```python
from build123d import *

# Parameters (mm, degrees)
SKETCH1_W                                  = 100
SKETCH1_H                                  = 100
BOSS_EXTRUDE1_DEPTH                        = 15
SKETCH2_R                                  = 0.5
CUT_EXTRUDE1_DEPTH                         = 2
MIRROR1_AT_THE_SECOND_PLANE_COPY_1_SKETC_R = 0.5
MIRROR1_AT_THE_SECOND_PLANE_COPY_1_DEPTH   = 2


with BuildPart() as part:
    # Sketch1 → Boss-Extrude1 (new body, symmetric)
    with BuildSketch(Plane(origin=(0, 0, 0), x_dir=(1, 0, 0), z_dir=(0, 1, 0))):
        Rectangle(SKETCH1_W, SKETCH1_H)
    extrude(amount=BOSS_EXTRUDE1_DEPTH, both=True)

    # Sketch2 → Cut-Extrude1 (cut)
    with BuildSketch(Plane(origin=(0, 15, 0), x_dir=(1, 0, 0), z_dir=(0, 1, 0))):
        Circle(SKETCH2_R)
        with BuildLine():
            Line((-28.090825198, -33.465171233), (-27.090825198, -33.120843619))
            ThreePointArc((-27.090825198, -33.120843619), (-25.819738468, -33.740794041), (-26.439688889, -35.011880771))
            Line((-26.439688889, -35.011880771), (-27.439688889, -35.356208384))
            ThreePointArc((-27.439688889, -35.356208384), (-28.710775619, -34.736257963), (-28.090825198, -33.465171233))
        make_face()
    cut_extrude1 = extrude(amount=-CUT_EXTRUDE1_DEPTH, mode=Mode.SUBTRACT)

    # Mirror1: Cut-Extrude1 across plane
    add(cut_extrude1.mirror(Plane.XY), mode=Mode.SUBTRACT)

    # Mirror1 at the second plane: Cut-Extrude1 across plane
    add(cut_extrude1.mirror(Plane(origin=(0, 0, 0), x_dir=(0, 0, 1), z_dir=(1, 0, 0))), mode=Mode.SUBTRACT)

    # Mirror1 at the second plane copy 1 sketc → Mirror1 at the second plane copy 1 (cut)
    with BuildSketch(Plane(origin=(0, 15, 0), x_dir=(-1, 0, 0), z_dir=(0, 1, 0))):
        Circle(MIRROR1_AT_THE_SECOND_PLANE_COPY_1_SKETC_R)
        with BuildLine():
            Line((-28.090825198, -33.465171233), (-27.090825198, -33.120843619))
            ThreePointArc((-27.090825198, -33.120843619), (-25.819738468, -33.740794041), (-26.439688889, -35.011880771))
            Line((-26.439688889, -35.011880771), (-27.439688889, -35.356208384))
            ThreePointArc((-27.439688889, -35.356208384), (-28.710775619, -34.736257963), (-28.090825198, -33.465171233))
        make_face()
    extrude(amount=-MIRROR1_AT_THE_SECOND_PLANE_COPY_1_DEPTH, mode=Mode.SUBTRACT)


solid = part.part
```
Source: CAD feature listing. Evaluate the final solid. Frame: model axes, mm. A direction names the side the tool comes from. Coordinates: 2 decimals unless noted, no trailing zeros. Put each result on its own line as item: value. Start each with the question number.
1) Reachability of faces 1 (the face through (-1, 15, -1)), 2 (the face through (27, 13, -34)) from +Z, -Z, +X, -X, +Y, -Y: full face, straight path, thin tool, end or side. Return the list, or none.
2) Contact query for a flat-ended pin moving along its axis: pin 1 Ø0.7 at (x, z) = (27.5, 34) entering from +Y. Output: stop coordinate, or through.
3) Ray query, L1, parallel to Z at x = 0, y = 13.9. Return the intervals inside material, ascending. Write a range as from..to.
4) Pull-direction query (Z, two-part tool) for faces 3 (the face through (-27, 13, 34)), 4 (the face through (27, 13, 34)), 5 (the face through (-1, 0, 50)), 6 (the face through (-1, 0, -50)); classes: pulls with the +Z half, pulls with the -Z half, needs draft (parallel to the pull), parting line crosses it, or undercut.
The answers:
1. face 1: +Z, -Z, +X, -X, +Y
1. face 2: +Y
2. pin 1: stops at y = 13
3. L1: z = -50..-0.5, 0.5..50
4. face 3: undercut
4. face 4: undercut
4. face 5: pulls with the +Z half
4. face 6: pulls with the -Z half
